For this review, take the finished solid that the model builds, in its own axes (mm). A direction names the side the tool comes from. Coordinates: 2 decimals unless noted, no trailing zeros. Loops run counter-clockwise (first coordinate to the right, second up) from the corner with the lowest first, then second, coordinate; pieces in that order, holes last. Notation, with made-up numbers: (29.25, -18) - (51.25, -18) arc R6 cw to (51.25, -13) - close; hole circle Ø8 at (-10, -39.75). An arc over 180 degrees is marked (long way). One line per item, written item: value. Start each with the question number.
1. For faces 5 (the face through (-17.15, 69.04, 51.99)), 6 (the face through (-16.7, 11.07, 33.5)), list the 3-axis set-ups (+Z, -Z, +X, -X, +Y, -Y) from which the entire face can be reached by the end or side of a thin tool; tool diameter is ignored.
2. Take a section at A-A, the plane x = -7.8. State the section outline as (y, z) points, and give its area (3 significant figures).
3. The part is to be moulded in two halves that separate along X. For faces 1 (the face through (-10, 71.5, 27)), 2 (the face through (-8.37, 69.04, 51.77)), 3 (the face through (-9.264, 69.035, 31.958)), 4 (the face through (-2.85, 69.04, 51.99)), say which applies: released by +X, released by -X, zero draft, split by the parting line, or undercut.
4. Take a section at B-B, the plane x = -14.75. State the section outline as (y, z) points.
5. To check wall thickness, follow line 1 (Y direction, x = -16, z = 15.5); line 2 (Y direction, x = -15, z = 32.5); line 3 (Y direction, x = -7, z = 28.5). State the ranges of each line that lie inside material, in increasing order. Write a range as from..to.
6. Take a section at D-D, the plane x = -1.5. State the section outline as (y, z) points.
7. Take a section at C-C, the plane y = -33.5. State the section outline as (x, z) points, and give its area (3 significant figures).
8. Insertion check: pin 1 (5 mm diameter, centred on x = -15.5, y = -2, fed in from +Z); pin 2 (6 mm diameter, centred on x = -14, y = 19.5, fed in from +Z). Each pin has a flat end and moves straight along its axis. Give the tip position at first contact, or say it passes through.
```python
from build123d import *

# Parameters (mm, degrees)
SKETCH1_W           = 20
SKETCH1_H           = 143
BOSS_EXTRUDE1_DEPTH = 10
SKETCH2_W           = 20
SKETCH2_H           = 5
BOSS_EXTRUDE2_DEPTH = 45
FILLET1_R           = 10
SKETCH6_R           = 1.5
CUT_EXTRUDE1_DEPTH  = 155.512135446
SKETCH2_3_W         = 6.51
SKETCH2_3_H         = 12.5
BOSS_EXTRUDE3_DEPTH = 25
FILLET2_R           = 5


with BuildPart() as part:
    # Sketch1 → Boss-Extrude1 (new body)
    with BuildSketch(Plane.XY):
        with Locations((-10, 0)):
            Rectangle(SKETCH1_W, SKETCH1_H)
    extrude(amount=BOSS_EXTRUDE1_DEPTH)

    # Sketch2 → Boss-Extrude2 (add)
    with BuildSketch(Plane.XY.offset(10)):
        with Locations((-10, 69)):
            Rectangle(SKETCH2_W, SKETCH2_H)
        with Locations((-10, -69)):
            Rectangle(SKETCH2_W, SKETCH2_H)
    extrude(amount=BOSS_EXTRUDE2_DEPTH)

    # Fillet1
    fillet1_edges = [part.edges().sort_by_distance(p)[0] for p in [
        (-20, -69, 55),
        (0, -69, 55),
        (-20, 69, 55),
        (0, 69, 55),
    ]]
    fillet(fillet1_edges, radius=FILLET1_R - 0.0001)  # a hair under: the kernel refuses the full size

    # Sketch6 → Cut-Extrude1 (cut, through all)
    with BuildSketch(Plane(origin=(0, 71.5, 0), x_dir=(1, 0, 0), z_dir=(0, 1, 0))):
        with Locations(Location((-7.8, -32.283583697, 0), (0, 0, 270))):
            Circle(SKETCH6_R)
        with Locations(Location((-7.8, -50.383583697, 0), (0, 0, 270))):
            Circle(SKETCH6_R)
    extrude(amount=-CUT_EXTRUDE1_DEPTH, mode=Mode.SUBTRACT)

    # Sketch2<3> → Boss-Extrude3 (add)
    with BuildSketch(Plane.XY.offset(10)):
        with Locations((-16.745, -6.25)):
            Rectangle(SKETCH2_3_W, SKETCH2_3_H)
        with Locations((-16.745, 6.25)):
            Rectangle(SKETCH2_3_W, SKETCH2_3_H)
    extrude(amount=BOSS_EXTRUDE3_DEPTH)

    # Fillet2
    fillet2_edges = [part.edges().sort_by_distance(p)[0] for p in [
        (-16.745, -12.5, 35),
        (-16.745, 12.5, 35),
    ]]
    fillet(fillet2_edges, radius=FILLET2_R)


solid = part.part
```
Solutions:
1. face 5: +Z, -X, +Y, -Y
1. face 6: +Z, +X, -X
2. outline: (-71.5, 0) - (71.5, 0) - (71.5, 30.78) - (66.5, 30.78) - (66.5, 10) - (-66.5, 10) - (-66.5, 30.78) - (-71.5, 30.78) - close; (-71.5, 33.78) - (-66.5, 33.78) - (-66.5, 48.88) - (-71.5, 48.88) - close; (-71.5, 51.88) - (-66.5, 51.88) - (-66.5, 54.76) - (-71.5, 54.76) - close; (66.5, 33.78) - (71.5, 33.78) - (71.5, 48.88) - (66.5, 48.88) - close; (66.5, 51.88) - (71.5, 51.88) - (71.5, 54.76) - (66.5, 54.76) - close
2. area: 1,820 mm2
3. face 1: zero draft
3. face 2: undercut
3. face 3: undercut
3. face 4: released by +X
4. outline: (-71.5, 0) - (71.5, 0) - (71.5, 53.8) - (66.5, 53.8) - (66.5, 10) - (12.5, 10) - (12.5, 30) arc R5 ccw to (7.5, 35) - (-7.5, 35) arc R5 ccw to (-12.5, 30) - (-12.5, 10) - (-66.5, 10) - (-66.5, 53.8) - (-71.5, 53.8) - close
5. line 1: -71.5..-66.5, -12.5..12.5, 66.5..71.5
5. line 2: -71.5..-66.5, -11.83..11.83, 66.5..71.5
5. line 3: -71.5..-66.5, 66.5..71.5
6. outline: (-71.5, 0) - (71.5, 0) - (71.5, 50.27) - (66.5, 50.27) - (66.5, 10) - (-66.5, 10) - (-66.5, 50.27) - (-71.5, 50.27) - close
7. outline: (-20, 0) - (0, 0) - (0, 10) - (-20, 10) - close
7. area: 200 mm2
8. pin 1: z = 35
8. pin 2: z = 10
